from build123d import *

# Parameters (mm, degrees)
SKETCH_R          = 6.6
PAD_DEPTH         = 30
COPYSKETCH001_R   = 17.5
COPYSKETCH001_R_2 = 6.6
PAD001_DEPTH      = 2
FILLET_R          = 1.9


with BuildPart() as part:
    # Sketch → Pad (new body)
    with BuildSketch(Plane.XY):
        Polygon((15.75, 0), (4.867018, 14.97914), (-12.742018, 9.257618), (-12.742018, -9.257618), (4.867018, -14.97914), align=None)
        Circle(SKETCH_R, mode=Mode.SUBTRACT)
    extrude(amount=PAD_DEPTH)

    # CopySketch001 → Pad001 (join)
    with BuildSketch(Plane(origin=(0, 0, 0), x_dir=(1, 0, 0), z_dir=(0, 0, -1))):
        Circle(COPYSKETCH001_R)
        Circle(COPYSKETCH001_R_2, mode=Mode.SUBTRACT)
    extrude(amount=PAD001_DEPTH)

    # Fillet
    fillet_edges = [part.edges().sort_by_distance(p)[0] for p in [
        (10.308509, 7.48957, 30),
        (-3.9375, 12.118379, 30),
        (-12.742018, 0, 30),
        (-3.9375, -12.118379, 30),
        (10.308509, -7.48957, 30),
        (-6.6, 0, 30),
        (-17.5, 0, -2),
    ]]
    fillet(fillet_edges, radius=FILLET_R)


solid = part.part
Geometry check sheet. Reference: the model listing, model coordinates, mm. A direction names the side the tool comes from. Give positions to 0.01 mm unless a question says otherwise; leave off trailing zeros. Loops run counter-clockwise (first coordinate to the right, second up) from the corner with the lowest first, then second, coordinate; pieces in that order, holes last. Notation, with made-up numbers: M 22,50 L 38,50 A28 cw 38,73 Z; hole C 45,-7 d2. An arc over 180 degrees is marked long. Answer as a JSON object with one key per item and string values. Group by question number.
Item 1: Access from +Z, -Z, +X, -X, +Y, -Y to the whole of each face (thin tool, end or side, straight path). Record for faces 1 (the flat face through (-4.06, -12.08, 13.85)), 2 (the flat face through (-3.81, 12.16, 13.85)), 3 (the flat face through (10.385, 7.385, 13.853)).
Item 2: Material ranges on L1, parallel to X at y = 0, z = 21; L2, parallel to Z at x = 9, y = 13; L3, parallel to X at y = -4, z = 12, recorded low to high.
Item 3: Gauge pin test, flat ends, axial feed: pin 1 (2 mm diameter, centred on x = 14, y = 13.5, fed in from +Z); pin 2 (2 mm diameter, centred on y = -11.5, z = 9, fed in from +X); pin 3 (12 mm diameter, centred on y = 1, z = 18.5, fed in from -X); pin 4 (4 mm diameter, centred on x = 3, z = 3, fed in from -Y). Record the tip position at first contact, or that the pin passes through.
Item 4: Sectioned sample at A-A on z = 2. Record the boundary of the cut face in (x, y), plus the area to 3 significant figures.
Findings below:
{
 "1": {"face 1": "+Z, -X, -Y", "face 2": "+Z, -X, +Y", "face 3": "+Z, +X, +Y"},
 "2": {"L1": "-12.74 to -6.6, 6.6 to 15.75", "L2": "-1.99 to 0", "L3": "-12.74 to -5.25, 5.25 to 12.84"},
 "3": {"pin 1": "through", "pin 2": "x = 8.12", "pin 3": "x = -12.74", "pin 4": "y = -14.98"},
 "4": {"outline": "M -12.74,-9.26 L 4.87,-14.98 L 15.75,0 L 4.87,14.98 L -12.74,9.26 Z; hole C 0,0 d13.2", "area": "453 mm2"}
}
